Design review of the part built by this model. Coordinates are the model's own, in mm. Face numbers are marked on the shaded views. A direction names the side the tool comes from. Round coordinates to 2 decimals unless told otherwise and drop trailing zeros. Loops run counter-clockwise (first coordinate to the right, second up) from the corner with the lowest first, then second, coordinate; pieces in that order, holes last. Notation, with made-up numbers: (55.25, 61) - (94.25, 61) arc R26 cw to (94.25, 77) - close; hole circle Ø8 at (86.25, 47). An arc over 180 degrees is marked (long way). Return JSON: item names as keys, results as strings. Group by question number.
(1) We need section C-C, the plane z = 252. Write out the cut boundary in (x, y).
(2) The part is to be moulded in two halves that separate along Z. For the marked faces 1, 2, 3 and 4, say which applies: pulls with the +Z half, pulls with the -Z half, needs draft (parallel to the pull), parting line crosses it, or undercut.
(3) Clearance check with flat-ended pins moving along their axes: pin 1 (5 mm diameter, centred on y = -41, z = 199, fed in from -X); pin 2 (5 mm diameter, centred on x = 6.5, z = 109, fed in from -Y); pin 3 (1.3 mm diameter, centred on y = 43, z = 137.5, fed in from -X). State where each tip first meets the part, or that it passes through.
(4) Wall thickness on L1, parallel to Y at x = 1, z = 71; L2, parallel to Z at x = -7.5, y = 43; L3, parallel to Y at x = -5.5, z = 246.5: over which ranges is each line inside the solid? List them lowest first. Write a range as [from, to].
(5) We need section A-A, the plane y = 0. Write out the cut boundary in (x, z).
(6) We need section D-D, the plane y = -31. Write out the cut boundary in (x, z).
(7) For the marked faces 5, 6, 7 and 8, list the 3-axis set-ups (+Z, -Z, +X, -X, +Y, -Y) from which the entire face can be reached by the end or side of a thin tool; tool diameter is ignored.
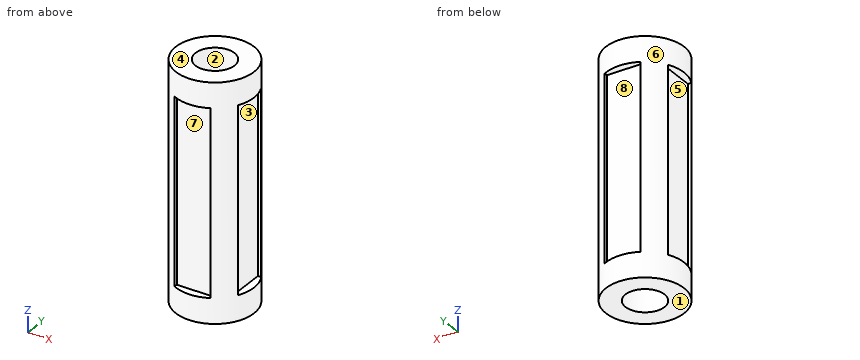
from build123d import *

# Parameters (mm, degrees)
SKETCH1_R           = 50
SKETCH1_R_2         = 25
BOSS_EXTRUDE1_DEPTH = 300
CUT_EXTRUDE1_DEPTH  = 10
CIRPATTERN1_COUNT   = 4


with BuildPart() as part:
    # Sketch1 → Boss-Extrude1 (new body)
    with BuildSketch(Plane.XY):
        Circle(SKETCH1_R)
        Circle(SKETCH1_R_2, mode=Mode.SUBTRACT)
    extrude(amount=BOSS_EXTRUDE1_DEPTH)

    # Sketch2 → Cut-Extrude1 (cut)
    with BuildSketch(Plane(origin=(0, 50, 0), x_dir=(1, 0, 0), z_dir=(0, 1, 0))):
        Polygon((-22.999966335, -268), (-22.995993926, -32), (22.995993926, -32), (22.999966335, -268), align=None)
    cut_extrude1 = extrude(amount=-CUT_EXTRUDE1_DEPTH, mode=Mode.SUBTRACT)

    # CirPattern1: Cut-Extrude1 ×4 about axis
    cirpattern1_axis = Axis((0, 0, 0), (0, 0, 1))
    for i in range(1, CIRPATTERN1_COUNT):
        add(cut_extrude1.rotate(cirpattern1_axis, i * 360 / CIRPATTERN1_COUNT), mode=Mode.SUBTRACT)


solid = part.part
Solutions:
{
 "1": {"outline": "(-44.4, -23) arc R50 ccw to (-23, -44.4) - (-23, -40) - (23, -40) - (23, -44.4) arc R50 ccw to (44.4, -23) - (40, -23) - (40, 23) - (44.4, 23) arc R50 ccw to (23, 44.4) - (23, 40) - (-23, 40) - (-23, 44.4) arc R50 ccw to (-44.4, 23) - (-40, 23) - (-40, -23) - close; hole circle Ø50 at (0, 0)"},
 "2": {"face 1": "pulls with the -Z half", "face 2": "needs draft", "face 3": "undercut", "face 4": "pulls with the +Z half"},
 "3": {"pin 1": "x = -31.9", "pin 2": "y = -40", "pin 3": "x = -26.58"},
 "4": {"L1": "[-40, -24.98], [24.98, 40]", "L2": "[0, 32], [268, 300]", "L3": "[-40, -24.39], [24.39, 40]"},
 "5": {"outline": "(-50, 0) - (-25, 0) - (-25, 300) - (-50, 300) - (-50, 268) - (-40, 268) - (-40, 32) - (-50, 32) - close; (25, 0) - (50, 0) - (50, 32) - (40, 32) - (40, 268) - (50, 268) - (50, 300) - (25, 300) - close"},
 "6": {"outline": "(-39.23, 0) - (39.23, 0) - (39.23, 300) - (-39.23, 300) - close"},
 "7": {"face 5": "-X", "face 6": "+Z, -Z", "face 7": "-Y", "face 8": "+Y"}
}
